For this review, take the finished solid that the model builds, in its own axes (mm). A direction names the side the tool comes from. Round coordinates to 2 decimals unless told otherwise and drop trailing zeros. Write each loop counter-clockwise with the first axis right and the second up, starting at its lowest first coordinate (ties: lowest second). Pieces come first, ordered by that corner, then holes. Notation, with made-up numbers: (62, 18.5) -> (87, 18.5) arc R15 ccw to (87, 38.5) -> close; hole circle Ø11 at (-8.75, 15.25). An arc over 180 degrees is marked (long way). Write each question's results on one line, items separated by ' | '. Start each with the question number.
Item 1: To check wall thickness, follow line 1 along Z through (x, y) = (-41, 3.2); line 2 along Z through (x, y) = (-21.5, 3.05); line 3 along X through (y, z) = (1.3, 34.5). State the ranges of each line that lie inside material, in increasing order.
Item 2: Add section B-B (z = 0). State the section outline as (x, y) points, plus the area to 3 significant figures.
Item 3: Add section D-D (x = -59). State the section outline as (y, z) points, plus the area to 3 significant figures.
Item 4: Add section A-A (y = 1.9). State the section outline as (x, z) points.
Item 5: Add section C-C (z = -58). State the section outline as (x, y) points.
Item 6: Clearance check with flat-ended pins moving along their axes: pin 1 (2 mm diameter, centred on x = -29, y = 3.5, fed in from +Z); pin 2 (1.5 mm diameter, centred on y = 2, z = -0.5, fed in from -X); pin 3 (2.5 mm diameter, centred on x = -48, y = 3.5, fed in from +Z). State where each tip first meets the part, or that it passes through.
Item 7: The part is to be moulded in two halves that separate along Z. For faces 1 (the flat face through (-48, 2, 5)), 2 (the cylindrical face through (-69.983, 2.465, 1.539)), 3 (the flat face through (-27, 5, -1)), say which applies: +Z half, -Z half, draft (parallel to the pull), parting line (faces both ways), or undercut.
Item 8: Tool access review of faces 4 (the flat face through (0, 2, -1)), 5 (the flat face through (-42.4, 3, 0)): name each direction out of +Z, -Z, +X, -X, +Y, -Y from which nothing blocks a thin tool from reaching the whole face with its end or side.
from build123d import *

# Parameters (mm, degrees)
SKETCH1_W           = 5
SKETCH1_H           = 10
BOSS_EXTRUDE1_DEPTH = 5
CUT_EXTRUDE1_DEPTH  = 10


with BuildPart() as part:
    # Sketch1 → Boss-Extrude1 (new body)
    with BuildSketch(Plane(origin=(0, 0, 0), x_dir=(1, 0, 0), z_dir=(0, 1, 0))):
        with BuildLine():
            Line((0, 70), (0, -70))
            ThreePointArc((0, -70), (-70, 0), (0, 70))
        make_face()
        with Locations((-47.5, 0)):
            Rectangle(SKETCH1_W, SKETCH1_H, mode=Mode.SUBTRACT)
    extrude(amount=BOSS_EXTRUDE1_DEPTH)

    # Sketch2 → Cut-Extrude1 (cut)
    with BuildSketch(Plane(origin=(0, 5, 0), x_dir=(1, 0, 0), z_dir=(0, 1, 0))):
        Polygon((-37.4, 0), (-37.4, -10), (-42.4, -10), (-42.4, 10), (-37.4, 10), align=None)
    extrude(amount=-CUT_EXTRUDE1_DEPTH, mode=Mode.SUBTRACT)


solid = part.part
Responses:
1) line 1: z = -56.74 to -10, 10 to 56.74 | line 2: z = -66.62 to 66.62 | line 3: x = -60.91 to 0
2) outline: (-70, 0) -> (-50, 0) -> (-50, 5) -> (-70, 5) -> close; (-45, 0) -> (-42.4, 0) -> (-42.4, 5) -> (-45, 5) -> close; (-37.4, 0) -> (0, 0) -> (0, 5) -> (-37.4, 5) -> close | area: 300 mm^2
3) outline: (0, -37.67) -> (5, -37.67) -> (5, 37.67) -> (0, 37.67) -> close | area: 377 mm^2
4) outline: (0, -70) -> (0, 70) arc R70 ccw to start; hole (-50, -5) -> (-45, -5) -> (-45, 5) -> (-50, 5) -> close; hole (-42.4, -10) -> (-37.4, -10) -> (-37.4, 10) -> (-42.4, 10) -> close
5) outline: (-39.19, 0) -> (0, 0) -> (0, 5) -> (-39.19, 5) -> close
6) pin 1: stops at z = 64.16 | pin 2: stops at x = -70 | pin 3: stops at z = 52.1
7) face 1: undercut | face 2: parting line | face 3: draft
8) face 4: +Z, -Z, +X, +Y, -Y | face 5: +Y, -Y
